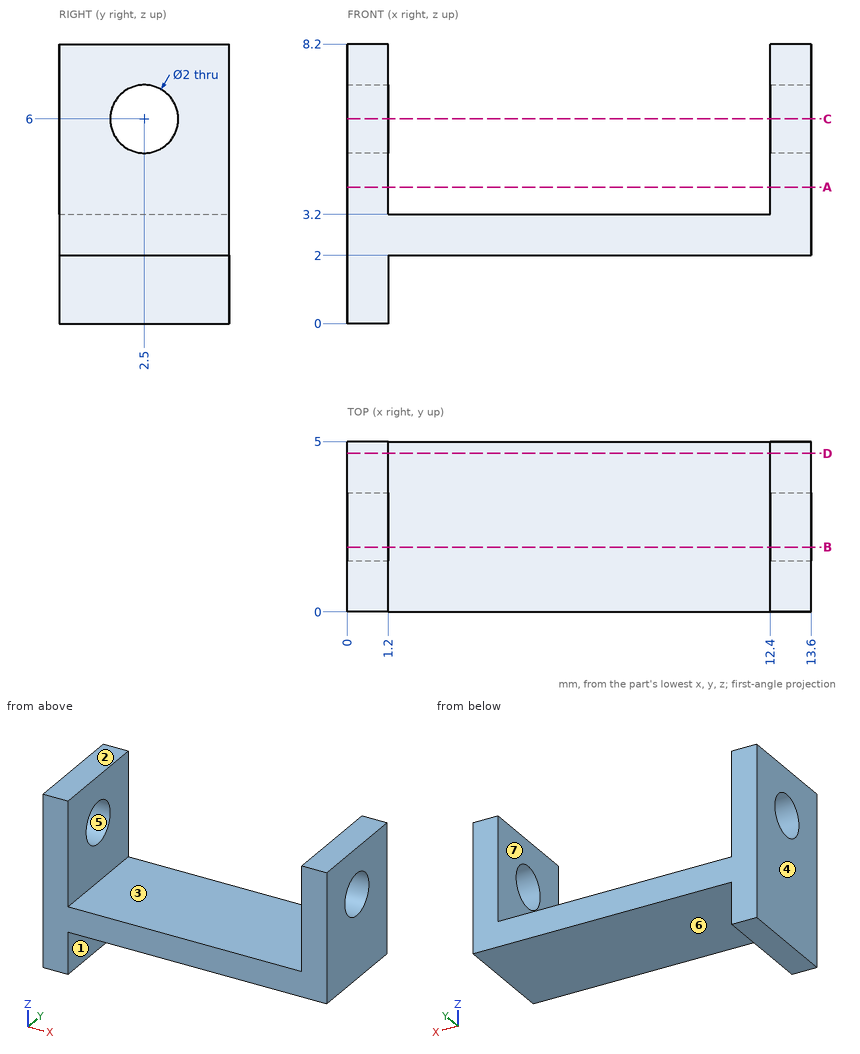
The drawing under review shows one solid part. Ordinate dimensions are in mm from its lowest x, y, z. A direction names the side the tool comes from. Coordinates: 2 decimals unless noted, no trailing zeros. Write each loop counter-clockwise with the first axis right and the second up, starting at its lowest first coordinate (ties: lowest second). Pieces come first, ordered by that corner, then holes. Notation, with made-up numbers: (-1.5, 33) - (14.5, 33) arc R28 cw to (14.5, 51) - close; hole circle Ø6 at (43, 86.25). An arc over 180 degrees is marked (long way). Answer as CSV lines item,"result".
(1) We need section B-B (y = 1.9). Give the boundary of the cut face in (x, z).
Data:
outline,"(0, 0) - (1.2, 0) - (1.2, 2) - (13.6, 2) - (13.6, 5.2) - (12.4, 5.2) - (12.4, 3.2) - (1.2, 3.2) - (1.2, 5.2) - (0, 5.2) - close; (0, 6.8) - (1.2, 6.8) - (1.2, 8.2) - (0, 8.2) - close; (12.4, 6.8) - (13.6, 6.8) - (13.6, 8.2) - (12.4, 8.2) - close"
(2) We need section D-D (y = 4.65). Give the boundary of the cut face in (x, z).
Data:
outline,"(0, 0) - (1.2, 0) - (1.2, 2) - (13.6, 2) - (13.6, 8.2) - (12.4, 8.2) - (12.4, 3.2) - (1.2, 3.2) - (1.2, 8.2) - (0, 8.2) - close"
(3) Clearance check with flat-ended pins moving along their axes: pin 1 Ø1 at (x, z) = (4.5, 5) entering from +Y; pin 2 Ø1 at (y, z) = (3, 0.5) entering from +X; pin 3 Ø1.5 at (x, y) = (5.5, 1.5) entering from -Z; pin 4 Ø3 at (x, y) = (5, 4.5) entering from +Z. State where each tip first meets the part, or that it passes through.
Data:
pin 1,"passes through"
pin 2,"stops at x = 1.2"
pin 3,"stops at z = 2"
pin 4,"stops at z = 3.2"
(4) We need section C-C (z = 6). Give the boundary of the cut face in (x, y).
Data:
outline,"(0, 0) - (1.2, 0) - (1.2, 1.5) - (0, 1.5) - close; (0, 3.5) - (1.2, 3.5) - (1.2, 5) - (0, 5) - close; (12.4, 0) - (13.6, 0) - (13.6, 1.5) - (12.4, 1.5) - close; (12.4, 3.5) - (13.6, 3.5) - (13.6, 5) - (12.4, 5) - close"
(5) We need section A-A (z = 4). Give the boundary of the cut face in (x, y), plus the area to 3 significant figures.
Data:
outline,"(0, 0) - (1.2, 0) - (1.2, 5) - (0, 5) - close; (12.4, 0) - (13.6, 0) - (13.6, 5) - (12.4, 5) - close"
area,"12.0 mm2"
(6) For line 1 along X through (y, z) = (0.5, 4.5); line 2 along Y through (x, z) = (0.85, 6); line 3 along Z through (x, y) = (3, 0.45), list the stretches that pass through material, from the lowest coordinate up. Write a range as [from, to].
Data:
line 1,"x = [0, 1.2], [12.4, 13.6]"
line 2,"y = [0, 1.5], [3.5, 5]"
line 3,"z = [2, 3.2]"
(7) Mouldability with a two-part tool opening along X and no side actions: class the marked faces 1, 2, 3 and 4 as pulls with the +X half, pulls with the -X half, needs draft (parallel to the pull), parting line crosses it, or undercut.
Data:
face 1,"pulls with the +X half"
face 2,"needs draft"
face 3,"undercut"
face 4,"pulls with the -X half"
(8) Tool access review of the marked faces 5, 6 and 7: name each direction out of +Z, -Z, +X, -X, +Y, -Y from which nothing blocks a thin tool from reaching the whole face with its end or side.
Data:
face 5,"+X, -X"
face 6,"-Z, +X, +Y, -Y"
face 7,"+Z, +Y, -Y"
